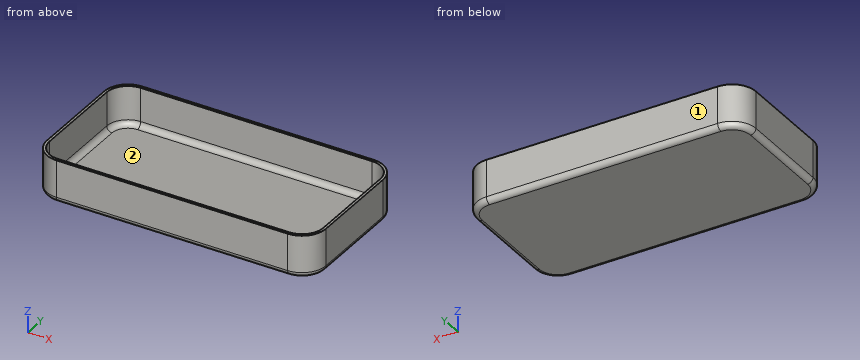
```python
from build123d import *

# Parameters (mm, degrees)
F0_W     = 52.8
F0_H     = 26.8
F0_W_2   = 51.8
F0_H_2   = 25.8
F1_DEPTH = 0.6
F2_DEPTH = 8
F3_R     = 4
F4_R     = 4.5
F5_R     = 1


with BuildPart() as f1:
    # F0 (on Top) → F1 (new body)
    with BuildSketch(Plane.XY):
        Rectangle(F0_W, F0_H)
        Rectangle(F0_W_2, F0_H_2, mode=Mode.SUBTRACT)
        Rectangle(F0_W_2, F0_H_2)
    extrude(amount=F1_DEPTH)

    # F0 (on Top) → F2 (join)
    with BuildSketch(Plane.XY):
        Rectangle(F0_W, F0_H)
        Rectangle(F0_W_2, F0_H_2, mode=Mode.SUBTRACT)
    extrude(amount=F2_DEPTH)

    # F3
    f3_edges = [f1.edges().sort_by_distance(p)[0] for p in [
        (-25.9, 12.9, 4.3),
        (25.9, 12.9, 4.3),
        (25.9, -12.9, 4.3),
        (-25.9, -12.9, 4.3),
    ]]
    fillet(f3_edges, radius=F3_R)

    # F4
    f4_edges = [f1.edges().sort_by_distance(p)[0] for p in [
        (26.4, 13.4, 4),
        (26.4, -13.4, 4),
        (-26.4, 13.4, 4),
        (-26.4, -13.4, 4),
    ]]
    fillet(f4_edges, radius=F4_R)

    # F5
    f5_edges = [f1.edges().sort_by_distance(p)[0] for p in [
        (0, 12.9, 0.6),
        (0, 13.4, 0),
    ]]
    fillet(f5_edges, radius=F5_R)


solid = f1.part
```
Check sheet for the modelled part. Datum: model origin and axes. Units: mm. Face numbers are marked on the shaded views. A direction names the side the tool comes from. Coordinates: 2 decimals unless noted, no trailing zeros. Loops run counter-clockwise (first coordinate to the right, second up) from the corner with the lowest first, then second, coordinate; pieces in that order, holes last.
1) Sectioned sample at B-B (y = -6.75). Record the boundary of the cut face in (x, z).
2) Access from +Z, -Z, +X, -X, +Y, -Y to the whole of each face (thin tool, end or side, straight path). Record for the marked faces 1 and 2.
3) Gauge pin test, flat ends, axial feed: pin 1 (5 mm diameter, centred on x = 13, y = -8.5, fed in from +Z); pin 2 (12 mm diameter, centred on x = 10, y = -8, fed in from +Z). Record the tip position at first contact, or that the pin passes through.
4) Material ranges on probe 1 along Y at (x, z) = (-14, 6); probe 2 along X at (y, z) = (1.75, 2.25); probe 3 along Z at (x, y) = (10.5, 4.5), recorded low to high.
5) Sectioned sample at A-A (z = 4.5). Record the boundary of the cut face in (x, y), and give its area (3 significant figures).
6) Sectioned sample at C-C (x = 21). Record the boundary of the cut face in (y, z).
Check sheet entries:
1. outline: (-26.4, 1) arc R1 ccw to (-25.4, 0) - (25.4, 0) arc R1 ccw to (26.4, 1) - (26.4, 8) - (25.9, 8) - (25.9, 1.6) arc R1 cw to (24.9, 0.6) - (-24.9, 0.6) arc R1 cw to (-25.9, 1.6) - (-25.9, 8) - (-26.4, 8) - close
2. face 1: +Z, -Z, +X, -X, +Y
2. face 2: +Z
3. pin 1: stops at z = 0.6
3. pin 2: stops at z = 8
4. probe 1: y = -13.4 to -12.9, 12.9 to 13.4
4. probe 2: x = -26.4 to -25.9, 25.9 to 26.4
4. probe 3: z = 0 to 0.6
5. outline: (-26.4, -8.9) arc R4.5 ccw to (-21.9, -13.4) - (21.9, -13.4) arc R4.5 ccw to (26.4, -8.9) - (26.4, 8.9) arc R4.5 ccw to (21.9, 13.4) - (-21.9, 13.4) arc R4.5 ccw to (-26.4, 8.9) - close; hole (-25.9, -8.9) arc R4 ccw to (-21.9, -12.9) - (21.9, -12.9) arc R4 ccw to (25.9, -8.9) - (25.9, 8.9) arc R4 ccw to (21.9, 12.9) - (-21.9, 12.9) arc R4 ccw to (-25.9, 8.9) - close
5. area: 75.0 mm2
6. outline: (-13.4, 1) arc R1 ccw to (-12.4, 0) - (12.4, 0) arc R1 ccw to (13.4, 1) - (13.4, 8) - (12.9, 8) - (12.9, 1.6) arc R1 cw to (11.9, 0.6) - (-11.9, 0.6) arc R1 cw to (-12.9, 1.6) - (-12.9, 8) - (-13.4, 8) - close
